For this review, use the dimensioned drawing (mm, ordinates from the lowest corner) and the shaded views. A direction names the side the tool comes from. Coordinates: 2 decimals unless noted, no trailing zeros. Write each loop counter-clockwise with the first axis right and the second up, starting at its lowest first coordinate (ties: lowest second). Pieces come first, ordered by that corner, then holes. Notation, with made-up numbers: M 89,-27.5 L 116,-27.5 A24 ccw 116,3.5 Z; hole C 51,53.5 d6. An arc over 180 degrees is marked long. Return JSON: item names as keys, results as strings.
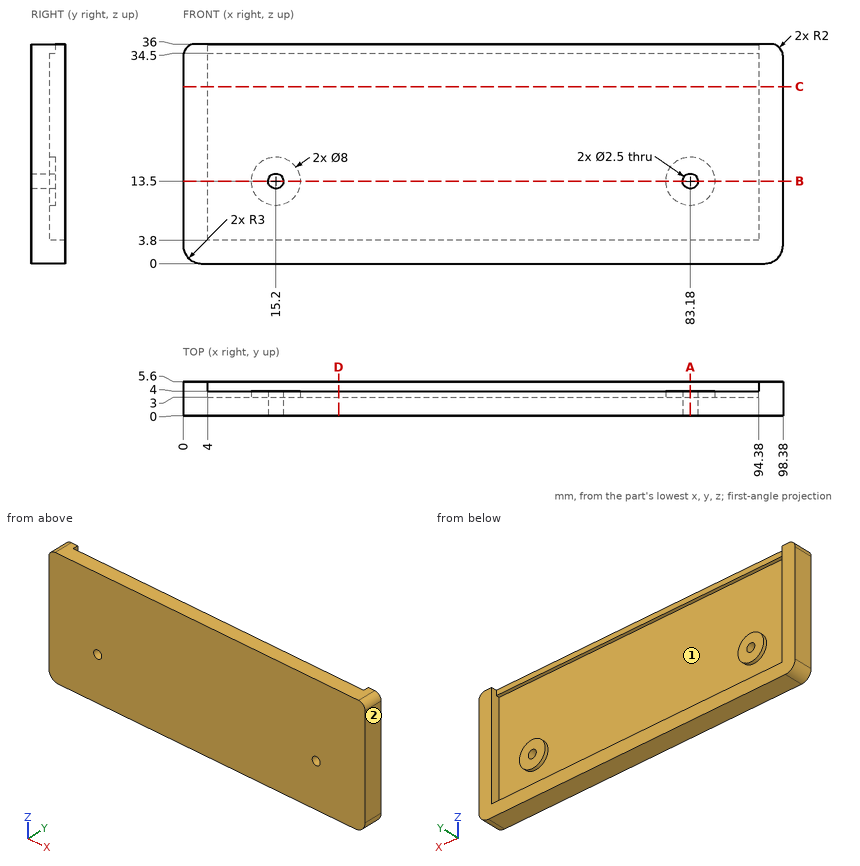
1. For the marked faces 1 and 2, list the 3-axis set-ups (+Z, -Z, +X, -X, +Y, -Y) from which the entire face can be reached by the end or side of a thin tool; tool diameter is ignored.
Checks:
{"face 1": "+Y", "face 2": "+Z, -Z, +X, +Y, -Y"}
2. We need section C-C (z = 29). State the section outline as (x, y) points, plus the area to 3 significant figures.
Checks:
{"outline": "M 0,0 L 98.38,0 L 98.38,5.6 L 94.38,5.6 L 94.38,3 L 4,3 L 4,5.6 L 0,5.6 Z", "area": "316 mm2"}
3. We need section D-D (x = 25.5). State the section outline as (y, z) points, plus the area to 3 significant figures.
Checks:
{"outline": "M 0,0 L 5.6,0 L 5.6,3.8 L 3,3.8 L 3,34.5 L 4,34.5 L 4,36 L 0,36 Z", "area": "119 mm2"}
4. We need section A-A (x = 83.18). State the section outline as (y, z) points, plus the area to 3 significant figures.
Checks:
{"outline": "M 0,0 L 5.6,0 L 5.6,3.8 L 3,3.8 L 3,9.5 L 4,9.5 L 4,12.25 L 0,12.25 Z; M 0,14.75 L 4,14.75 L 4,17.5 L 3,17.5 L 3,34.5 L 4,34.5 L 4,36 L 0,36 Z", "area": "117 mm2"}
5. Wall thickness on L1, parallel to X at y = 0.9, z = 13.5; L2, parallel to Z at x = 83.18, y = 2.2; L3, parallel to X at y = 3.6, z = 28: over which ranges is each line inside the solid? List them lowest first. Write a range as from..to.
Checks:
{"L1": "0..13.95, 16.45..81.93, 84.43..98.38", "L2": "0..12.25, 14.75..36", "L3": "0..4, 94.38..98.38"}
6. We need section B-B (z = 13.5). State the section outline as (x, y) points, plus the area to 3 significant figures.
Checks:
{"outline": "M 0,0 L 13.95,0 L 13.95,4 L 11.2,4 L 11.2,3 L 4,3 L 4,5.6 L 0,5.6 Z; M 16.45,0 L 81.93,0 L 81.93,4 L 79.18,4 L 79.18,3 L 19.2,3 L 19.2,4 L 16.45,4 Z; M 84.43,0 L 98.38,0 L 98.38,5.6 L 94.38,5.6 L 94.38,3 L 87.18,3 L 87.18,4 L 84.43,4 Z", "area": "312 mm2"}
7. Clearance check with flat-ended pins moving along their axes: pin 1 Ø12 at (x, z) = (69, 13) entering from +Y; pin 2 Ø0.8 at (x, z) = (57, 35) entering from +Y. State where each tip first meets the part, or that it passes through.
Checks:
{"pin 1": "y = 3", "pin 2": "y = 4"}
